Source: CAD feature listing. Evaluate the final solid. Frame: model axes, mm. Face numbers are marked on the shaded views. A direction names the side the tool comes from. Coordinates: 2 decimals unless noted, no trailing zeros. Write each loop counter-clockwise with the first axis right and the second up, starting at its lowest first coordinate (ties: lowest second). Pieces come first, ordered by that corner, then holes. Notation, with made-up numbers: (-36, 82.25) -> (14, 82.25) arc R27 ccw to (14, 119.25) -> close; hole circle Ø2 at (64, 58.25). An arc over 180 degrees is marked (long way). One line per item, written item: value. Start each with the question number.
1. Access query for the marked faces 1, 2 and 3. Directions: +Z, -Z, +X, -X, +Y, -Y. A direction counts if a zero-diameter tool reaches every point of the face in a straight line with its end or side. Return the directions, or none.
2. Section query A-A, the plane x = 0. Output: boundary loops of the cut face in (y, z).
3. First-contact query: P1, Ø5, axis at y = 10.5, z = -8.5, coming from the -X side; P2, Ø1.5, axis at x = -9.5, y = 9, coming from the -Z side; P3, Ø6, axis at x = -3.5, y = 7.5, coming from the +Z side. Flat tips, straight axial feed; report the tip coordinate or a pass-through.
4. Section query B-B, the plane z = 0. Output: boundary loops of the cut face in (x, y), and give its area (3 significant figures).
5. Line query: line 1 (Z direction, x = 0, y = 15.5); line 2 (Y direction, x = -5.5, z = 3). Output: solid intervals per line, ascending.
6. Section query C-C, the plane y = 2.25. Output: boundary loops of the cut face in (x, z), and give its area (3 significant figures).
from build123d import *

# Parameters (mm, degrees)
F0_R     = 15
F1_DEPTH = 20
F2_R     = 13
F3_DEPTH = 9
F4_R     = 13
F5_DEPTH = 9


with BuildPart() as f1:
    # F0 (on Front) → F1 (new body)
    with BuildSketch(Plane.XZ):
        Circle(F0_R)
    extrude(amount=-F1_DEPTH)

    # F2 (on face) → F3 (cut)
    with BuildSketch(Plane.XZ):
        Circle(F2_R)
    extrude(amount=-F3_DEPTH, mode=Mode.SUBTRACT)

    # F4 (on face) → F5 (cut)
    with BuildSketch(Plane(origin=(0, 20, 0), x_dir=(-1, 0, 0), z_dir=(0, 1, 0))):
        Circle(F4_R)
    extrude(amount=-F5_DEPTH, mode=Mode.SUBTRACT)


solid = f1.part
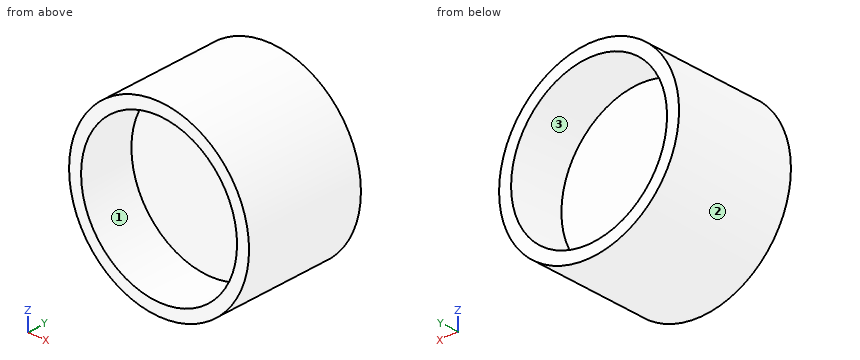
Computed values:
1. face 1: -Y
1. face 2: +Y, -Y
1. face 3: +Y
2. outline: (0, -15) -> (20, -15) -> (20, -13) -> (11, -13) -> (11, 13) -> (20, 13) -> (20, 15) -> (0, 15) -> (0, 13) -> (9, 13) -> (9, -13) -> (0, -13) -> close
3. P1: stops at x = -13.75
3. P2: stops at z = -12.18
3. P3: stops at z = 14.99
4. outline: (-15, 0) -> (-13, 0) -> (-13, 9) -> (13, 9) -> (13, 0) -> (15, 0) -> (15, 20) -> (13, 20) -> (13, 11) -> (-13, 11) -> (-13, 20) -> (-15, 20) -> close
4. area: 132 mm²
5. line 1: z = -15 to -13, 13 to 15
5. line 2: y = 9 to 11
6. outline: circle Ø30 at (0, 0); hole circle Ø26 at (0, 0)
6. area: 176 mm²
